```python
from build123d import *

# Parameters (mm, degrees)
EXTRUDE_1_DEPTH     = 2.5
SKETCH_4_R          = 4
CUT_EXTRUDE_1_DEPTH = 6
CHAMFER_1_SIZE      = 0.8
CHAMFER_2_SIZE      = 0.8


with BuildPart() as part:
    # 草图1 → 凸台-拉伸1 (new, symmetric)
    with BuildSketch(Plane(origin=(0, 0, 0), x_dir=(1, 0, 0), z_dir=(0, 1, 0))):
        with BuildLine():
            ThreePointArc((-9.860132972, 1.666666667), (-10, 0), (-9.860132972, -1.666666667))
            ThreePointArc((-9.860132972, -1.666666667), (-9.471702803, -2.301806962), (-8.752043547, -2.49252074))
            ThreePointArc((-8.752043547, -2.49252074), (-8.629852726, -2.486913493), (-8.50823537, -2.5))
            ThreePointArc((-8.50823537, -2.5), (-6.445172036, -2.661121156), (-4.394270374, -2.385453391))
            ThreePointArc((-4.394270374, -2.385453391), (-3.535533906, -3.535533906), (-2.385453391, -4.394270374))
            ThreePointArc((-2.385453391, -4.394270374), (-2.661121156, -6.445172036), (-2.5, -8.50823537))
            ThreePointArc((-2.5, -8.50823537), (-2.486913493, -8.629852726), (-2.49252074, -8.752043547))
            ThreePointArc((-2.49252074, -8.752043547), (-2.301806962, -9.471702803), (-1.666666667, -9.860132972))
            ThreePointArc((-1.666666667, -9.860132972), (0, -10), (1.666666667, -9.860132972))
            ThreePointArc((1.666666667, -9.860132972), (2.301806962, -9.471702803), (2.49252074, -8.752043547))
            ThreePointArc((2.49252074, -8.752043547), (2.486913493, -8.629852726), (2.5, -8.50823537))
            ThreePointArc((2.5, -8.50823537), (2.661121156, -6.445172036), (2.385453391, -4.394270374))
            ThreePointArc((2.385453391, -4.394270374), (3.535533906, -3.535533906), (4.394270374, -2.385453391))
            ThreePointArc((4.394270374, -2.385453391), (6.445172036, -2.661121156), (8.50823537, -2.5))
            ThreePointArc((8.50823537, -2.5), (8.629852726, -2.486913493), (8.752043547, -2.49252074))
            ThreePointArc((8.752043547, -2.49252074), (9.471702803, -2.301806962), (9.860132972, -1.666666667))
            ThreePointArc((9.860132972, -1.666666667), (10, 0), (9.860132972, 1.666666667))
            ThreePointArc((9.860132972, 1.666666667), (9.471702803, 2.301806962), (8.752043547, 2.49252074))
            ThreePointArc((8.752043547, 2.49252074), (8.629852726, 2.486913493), (8.50823537, 2.5))
            ThreePointArc((8.50823537, 2.5), (6.445172036, 2.661121156), (4.394270374, 2.385453391))
            ThreePointArc((4.394270374, 2.385453391), (3.535533906, 3.535533906), (2.385453391, 4.394270374))
            ThreePointArc((2.385453391, 4.394270374), (2.661121156, 6.445172036), (2.5, 8.50823537))
            ThreePointArc((2.5, 8.50823537), (2.486913493, 8.629852726), (2.49252074, 8.752043547))
            ThreePointArc((2.49252074, 8.752043547), (2.301806962, 9.471702803), (1.666666667, 9.860132972))
            ThreePointArc((1.666666667, 9.860132972), (0, 10), (-1.666666667, 9.860132972))
            ThreePointArc((-1.666666667, 9.860132972), (-2.301806962, 9.471702803), (-2.49252074, 8.752043547))
            ThreePointArc((-2.49252074, 8.752043547), (-2.486913493, 8.629852726), (-2.5, 8.50823537))
            ThreePointArc((-2.5, 8.50823537), (-2.661121156, 6.445172036), (-2.385453391, 4.394270374))
            ThreePointArc((-2.385453391, 4.394270374), (-3.535533906, 3.535533906), (-4.394270374, 2.385453391))
            ThreePointArc((-4.394270374, 2.385453391), (-6.445172036, 2.661121156), (-8.50823537, 2.5))
            ThreePointArc((-8.50823537, 2.5), (-8.629852726, 2.486913493), (-8.752043547, 2.49252074))
            ThreePointArc((-8.752043547, 2.49252074), (-9.471702803, 2.301806962), (-9.860132972, 1.666666667))
        make_face()
    extrude(amount=EXTRUDE_1_DEPTH, both=True)

    # 草图4 → 切除-拉伸1 (cut, symmetric)
    with BuildSketch(Plane(origin=(0, 2.5, 0), x_dir=(1, 0, 0), z_dir=(0, 1, 0))):
        with Locations(Location((0, 0, 0), (0, 0, 90))):
            Circle(SKETCH_4_R)
    extrude(amount=CUT_EXTRUDE_1_DEPTH, both=True, mode=Mode.SUBTRACT)

    # 倒角1
    chamfer_1_edges = [part.edges().sort_by_distance(p)[0] for p in [
        (0, 2.5, 4),
    ]]
    chamfer(chamfer_1_edges, length=CHAMFER_1_SIZE)

    # 倒角2
    chamfer_2_edges = [part.edges().sort_by_distance(p)[0] for p in [
        (0, -2.5, 4),
    ]]
    chamfer(chamfer_2_edges, length=CHAMFER_2_SIZE)


solid = part.part
```
Here's how the part is built. I have some questions about the finished solid (model axes, mm). Give positions to 0.01 mm unless a question says otherwise; leave off trailing zeros. Write each loop counter-clockwise with the first axis right and the second up, starting at its lowest first coordinate (ties: lowest second). Pieces come first, ordered by that corner, then holes. Notation, with made-up numbers: M -20,15 L 11,15 A13 ccw 11,28 Z; hole C 27,62.5 d10. An arc over 180 degrees is marked long. Put each result on its own line as item: value. Start each with the question number.
Item 1: Thinking about a two-plate mould opening in Z: for faces 1 (the cylindrical face through (0, 0, -10)), 2 (the cylindrical face through (6.42, 0.04, 2.66)), 3 (the cylindrical face through (-2.66, 0.04, -6.47)), which applies, +Z half, -Z half, draft (parallel to the pull), parting line (faces both ways), or undercut?
Item 2: Will this pin go through, and if not, where does the flat tip stop? pin 1 (1 mm diameter, centred on y = 1.5, z = 7.5, fed in from -X).
Item 3: If we section it at A-A, the plane z = 0: Write out the boundary of the cut face in (x, y), then the cut area to 3 significant figures.
Item 4: I need wall thicknesses on L1, parallel to Z at x = 3.5, y = 2.2; L2, parallel to Z at x = -3.25, y = 1.85; L3, parallel to X at y = -0.75, z = -2.25. Which ranges of each line are inside material? Lowest first, please. Write a range as from..to.
Item 5: If we section it at D-D, the plane x = -7.5: Write out the boundary of the cut face in (y, z).
Item 6: If we section it at B-B, the plane x = 0: Write out the boundary of the cut face in (y, z), then the cut area to 3 significant figures.
Values:
1. face 1: -Z half
1. face 2: +Z half
1. face 3: undercut
2. pin 1: x = -2.66
3. outline: M -10,-2.5 L -4.8,-2.5 L -4,-1.7 L -4,1.7 L -4.8,2.5 L -10,2.5 Z; M 4,-1.7 L 4.8,-2.5 L 10,-2.5 L 10,2.5 L 4.8,2.5 L 4,1.7 Z
3. area: 58.7 mm²
4. L1: -3.57..-2.83, 2.83..3.57
4. L2: -3.8..-2.58, 2.58..3.8
4. L3: -9.54..-3.31, 3.31..9.54
5. outline: M -2.5,-2.63 L 2.5,-2.63 L 2.5,2.63 L -2.5,2.63 Z
6. outline: M -2.5,-10 L 2.5,-10 L 2.5,-4.8 L 1.7,-4 L -1.7,-4 L -2.5,-4.8 Z; M -2.5,4.8 L -1.7,4 L 1.7,4 L 2.5,4.8 L 2.5,10 L -2.5,10 Z
6. area: 58.7 mm²
